Geometry check sheet. Reference: the model listing, model coordinates, mm. Face numbers are marked on the shaded views. A direction names the side the tool comes from. Give positions to 0.01 mm unless a question says otherwise; leave off trailing zeros. Loops run counter-clockwise (first coordinate to the right, second up) from the corner with the lowest first, then second, coordinate; pieces in that order, holes last. Notation, with made-up numbers: (59.5, 46.25) -> (71.5, 46.25) arc R32 cw to (71.5, 77.25) -> close; hole circle Ø3 at (-25, -18). An arc over 180 degrees is marked (long way). One line per item, written item: value. Start each with the question number.
(1) Scan lines: line 1 along Y through (x, z) = (691, -1421.5); line 2 along X through (y, z) = (1194, -1417.75); line 3 along Y through (x, z) = (725, -1423.25). Record each from-to range of solid material in increasing order. Write a range as from..to.
(2) Gauge pin test, flat ends, axial feed: pin 1 Ø5 at (x, y) = (726.5, 1160.5) entering from +Z; pin 2 Ø4 at (x, y) = (676.5, 1150.5) entering from -Z; pin 3 Ø2 at (y, z) = (1147.5, -1423) entering from -X. Record the tip position at first contact, or that the pin passes through.
(3) Sectioned sample at C-C, the plane x = 720. Record the cut outline in (y, z), then the cut area to 3 significant figures.
(4) Sectioned sample at B-B, the plane z = -1419.25. Record the cut outline in (x, y).
(5) Tool access check on the marked faces 1, 2 and 3. Record the directions out of +Z, -Z, +X, -X, +Y, -Y that give a thin tool (end or side, any length) a straight path to the whole face; none if there is none.
(6) Sectioned sample at A-A, the plane y = 1183.5. Record the cut outline in (x, z), then the cut area to 3 significant figures.
(7) Draft check along Y on the marked faces 4, 5, 6 and 7. Enter one of: pulls with the +Y half, pulls with the -Y half, needs draft (parallel to the pull), parting line crosses it, or undercut.
from build123d import *

# Parameters (mm, degrees)
BOSS_EXTRU_1_DEPTH = 7.5
ESQUISSE2_W        = 7.25
ESQUISSE2_H        = 7.25
BOSS_EXTRU_2_DEPTH = 4
CONG_1_R           = 2
CONG_2_R           = 0.5
BOSS_EXTRU_3_DEPTH = 1.6


with BuildPart() as part:
    # Esquisse1 → Boss.-Extru.1 (new body)
    with BuildSketch(Plane.XY.offset(-1424.691834437)):
        with BuildLine():
            Line((670.002412047, 1197.108127391), (670.002412047, 1149.108126022))
            ThreePointArc((670.002412047, 1149.108126022), (671.759771358, 1144.86548622), (676.002410874, 1143.108126218))
            Line((676.002410874, 1143.108126218), (727.002412047, 1143.108126218))
            ThreePointArc((727.002412047, 1143.108126218), (731.245051976, 1144.865485459), (733.002412047, 1149.108125045))
            Line((733.002412047, 1149.108125045), (733.002412047, 1197.108126218))
            ThreePointArc((733.002412047, 1197.108126218), (731.245052806, 1201.350766146), (727.00241322, 1203.108126218))
            Line((727.00241322, 1203.108126218), (676.00241121, 1203.108126218))
            ThreePointArc((676.00241121, 1203.108126218), (671.759771822, 1201.35076668), (670.002412047, 1197.108127391))
        make_face()
        with BuildLine():
            Line((676.002411852, 1145.608126218), (727.002412047, 1145.608126218))
            ThreePointArc((727.002412047, 1145.608126218), (729.477285369, 1146.633252758), (730.502412047, 1149.108126022))
            Line((730.502412047, 1149.108126022), (730.502412047, 1197.108126218))
            ThreePointArc((730.502412047, 1197.108126218), (729.477285507, 1199.582999539), (727.002412243, 1200.608126218))
            Line((727.002412243, 1200.608126218), (676.002412047, 1200.608126218))
            ThreePointArc((676.002412047, 1200.608126218), (673.527538726, 1199.582999677), (672.502412047, 1197.108126413))
            Line((672.502412047, 1197.108126413), (672.502412047, 1149.108126022))
            ThreePointArc((672.502412047, 1149.108126022), (673.527538657, 1146.633252827), (676.002411852, 1145.608126218))
        make_face(mode=Mode.SUBTRACT)
    extrude(amount=BOSS_EXTRU_1_DEPTH)

    # Esquisse2 → Boss.-Extru.2 (add)
    with BuildSketch(Plane(origin=(0, 0, -1424.691834437), x_dir=(1, 0, 0), z_dir=(0, 0, -1))):
        with Locations((676.127412047, -1149.233126218)):
            Rectangle(ESQUISSE2_W, ESQUISSE2_H)
        with Locations((726.877412243, -1149.233126218)):
            Rectangle(ESQUISSE2_W, ESQUISSE2_H)
        with Locations((726.877412243, -1196.983126022)):
            Rectangle(ESQUISSE2_W, ESQUISSE2_H)
        with Locations((676.127412047, -1196.983126022)):
            Rectangle(ESQUISSE2_W, ESQUISSE2_H)
    extrude(amount=-BOSS_EXTRU_2_DEPTH)

    # Cong_1
    cong_1_edges = [part.edges().sort_by_distance(p)[0] for p in [
        (679.752412047, 1152.858126218, -1422.691834437),
        (679.752412047, 1193.358126022, -1422.691834437),
        (723.252412243, 1193.358126022, -1422.691834437),
        (723.252412243, 1152.858126218, -1422.691834437),
    ]]
    fillet(cong_1_edges, radius=CONG_1_R)

    # Cong_2
    cong_2_edges = [part.edges().sort_by_distance(p)[0] for p in [
        (672.502412047, 1152.858126218, -1422.691834437),
        (679.752412047, 1145.608126218, -1422.691834437),
        (679.752412047, 1200.608126022, -1422.691834437),
        (672.502412047, 1193.358126022, -1422.691834437),
        (730.502412243, 1193.358126022, -1422.691834437),
        (723.252412243, 1200.608126022, -1422.691834437),
        (723.252412243, 1145.608126218, -1422.691834437),
        (730.502412243, 1152.858126218, -1422.691834437),
    ]]
    fillet(cong_2_edges, radius=CONG_2_R)

    # Esquisse1_2 → Boss.-Extru.3 (add)
    with BuildSketch(Plane.XY.offset(-1424.691834437)):
        with BuildLine():
            Line((670.002412047, 1197.108127391), (670.002412047, 1149.108126022))
            ThreePointArc((670.002412047, 1149.108126022), (671.759771358, 1144.86548622), (676.002410874, 1143.108126218))
            Line((676.002410874, 1143.108126218), (727.002412047, 1143.108126218))
            ThreePointArc((727.002412047, 1143.108126218), (731.245051976, 1144.865485459), (733.002412047, 1149.108125045))
            Line((733.002412047, 1149.108125045), (733.002412047, 1197.108126218))
            ThreePointArc((733.002412047, 1197.108126218), (731.245052806, 1201.350766146), (727.00241322, 1203.108126218))
            Line((727.00241322, 1203.108126218), (676.00241121, 1203.108126218))
            ThreePointArc((676.00241121, 1203.108126218), (671.759771822, 1201.35076668), (670.002412047, 1197.108127391))
        make_face()
        with BuildLine():
            Line((676.002411852, 1145.608126218), (727.002412047, 1145.608126218))
            ThreePointArc((727.002412047, 1145.608126218), (729.477285369, 1146.633252758), (730.502412047, 1149.108126022))
            Line((730.502412047, 1149.108126022), (730.502412047, 1197.108126218))
            ThreePointArc((730.502412047, 1197.108126218), (729.477285507, 1199.582999539), (727.002412243, 1200.608126218))
            Line((727.002412243, 1200.608126218), (676.002412047, 1200.608126218))
            ThreePointArc((676.002412047, 1200.608126218), (673.527538726, 1199.582999677), (672.502412047, 1197.108126413))
            Line((672.502412047, 1197.108126413), (672.502412047, 1149.108126022))
            ThreePointArc((672.502412047, 1149.108126022), (673.527538657, 1146.633252827), (676.002411852, 1145.608126218))
        make_face(mode=Mode.SUBTRACT)
    extrude(amount=-BOSS_EXTRU_3_DEPTH)


solid = part.part
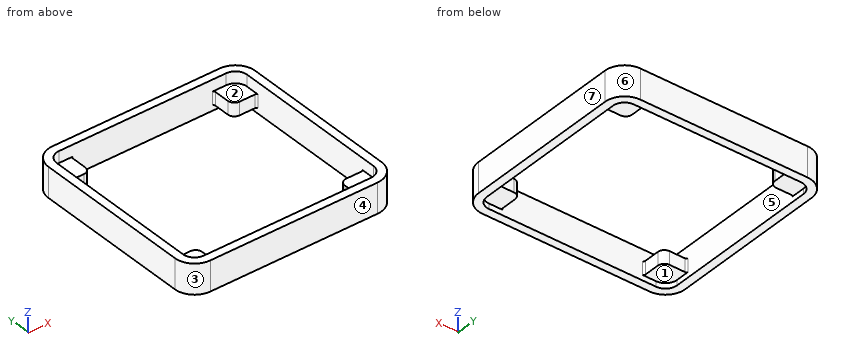
Calculated:
1. line 1: y = 1143.11..1145.61, 1200.61..1203.11
1. line 2: x = 670..672.5, 730.5..733
1. line 3: y = 1143.11..1152.84, 1193.37..1203.11
2. pin 1: passes through
2. pin 2: stops at z = -1424.69
2. pin 3: stops at x = 670.03
3. outline: (1143.11, -1426.29) -> (1145.61, -1426.29) -> (1145.61, -1417.19) -> (1143.11, -1417.19) -> close; (1200.61, -1426.29) -> (1203.11, -1426.29) -> (1203.11, -1417.19) -> (1200.61, -1417.19) -> close
3. area: 45.5 mm2
4. outline: (670, 1149.11) arc R6 ccw to (676, 1143.11) -> (727, 1143.11) arc R6 ccw to (733, 1149.11) -> (733, 1197.11) arc R6 ccw to (727, 1203.11) -> (676, 1203.11) arc R6 ccw to (670, 1197.11) -> close; hole (672.5, 1149.11) arc R3.5 ccw to (676, 1145.61) -> (727, 1145.61) arc R3.5 ccw to (730.5, 1149.11) -> (730.5, 1197.11) arc R3.5 ccw to (727, 1200.61) -> (676, 1200.61) arc R3.5 ccw to (672.5, 1197.11) -> close
5. face 1: -Z
5. face 2: +Z
5. face 3: +Z, -Z, -X, -Y
6. outline: (670, -1426.29) -> (672.5, -1426.29) -> (672.5, -1417.19) -> (670, -1417.19) -> close; (730.5, -1426.29) -> (733, -1426.29) -> (733, -1417.19) -> (730.5, -1417.19) -> close
6. area: 45.5 mm2
7. face 4: pulls with the -Y half
7. face 5: undercut
7. face 6: pulls with the +Y half
7. face 7: needs draft
